For this review, take the finished solid that the model builds, in its own axes (mm). Coordinates: 2 decimals unless noted, no trailing zeros. Loops run counter-clockwise (first coordinate to the right, second up) from the corner with the lowest first, then second, coordinate; pieces in that order, holes last. Notation, with made-up numbers: M 39.5,-31.75 L 50.5,-31.75 A29 cw 50.5,-6.75 Z; hole C 28.25,80 d8. An arc over 180 degrees is marked long. Answer as a JSON object with one key per item and string values. Group by question number.
Item 1: Add section B-B (x = 62). State the section outline as (y, z) points, then the cut area to 3 significant figures.
Item 2: Wall thickness on L1, parallel to X at y = 82, z = 2.8; L2, parallel to Y at x = 86, z = 2.6: over which ranges is each line inside the solid? List them lowest first. Write a range as from..to.
Item 3: Add section A-A (y = 84.5). State the section outline as (x, z) points.
Item 4: Add section C-C (z = 1.4). State the section outline as (x, y) points.
from build123d import *

# Parameters (mm, degrees)
BOX001_W     = 98
BOX001_H     = 174
BOX001_DEPTH = 10
FILLET_R     = 1.5
BOX_W        = 120
BOX_H        = 181
BOX_DEPTH    = 3
FILLET001_R  = 1.5


with BuildPart() as fillet_body:
    # Box001 → Box001 (new body)
    with BuildSketch(Plane(origin=(7, 3.5, 0), x_dir=(1, 0, 0), z_dir=(0, 0, 1))):
        with Locations((49, 87)):
            Rectangle(BOX001_W, BOX001_H)
    extrude(amount=BOX001_DEPTH)

    # Fillet
    fillet_edges = [fillet_body.edges().sort_by_distance(p)[0] for p in [
        (7, 3.5, 5),
        (7, 177.5, 5),
        (105, 3.5, 5),
        (105, 177.5, 5),
    ]]
    fillet(fillet_edges, radius=FILLET_R)


with BuildPart() as cut:
    # Box → Box (new body)
    with BuildSketch(Plane(origin=(2, 0, 0), x_dir=(1, 0, 0), z_dir=(0, 0, 1))):
        with Locations((60, 90.5)):
            Rectangle(BOX_W, BOX_H)
    extrude(amount=BOX_DEPTH)

    # Fillet001
    fillet001_edges = [cut.edges().sort_by_distance(p)[0] for p in [
        (2, 0, 1.5),
        (2, 181, 1.5),
        (122, 0, 1.5),
        (122, 181, 1.5),
    ]]
    fillet(fillet001_edges, radius=FILLET001_R)

    # Cut: cut Fillet body
    add(fillet_body.part, mode=Mode.SUBTRACT)


solid = cut.part
From the geometry:
{
 "1": {"outline": "M 0,0 L 3.5,0 L 3.5,3 L 0,3 Z; M 177.5,0 L 181,0 L 181,3 L 177.5,3 Z", "area": "21.0 mm²"},
 "2": {"L1": "x = 2..7, 105..122", "L2": "y = 0..3.5, 177.5..181"},
 "3": {"outline": "M 2,0 L 7,0 L 7,3 L 2,3 Z; M 105,0 L 122,0 L 122,3 L 105,3 Z"},
 "4": {"outline": "M 2,1.5 A1.5 ccw 3.5,0 L 120.5,0 A1.5 ccw 122,1.5 L 122,179.5 A1.5 ccw 120.5,181 L 3.5,181 A1.5 ccw 2,179.5 Z; hole M 7,5 A1.5 ccw 8.5,3.5 L 103.5,3.5 A1.5 ccw 105,5 L 105,176 A1.5 ccw 103.5,177.5 L 8.5,177.5 A1.5 ccw 7,176 Z"}
}
